from build123d import *

# Parameters (mm, degrees)
BOSS_EXTRUDE1_DEPTH = 114.3
SKETCH6_W           = 27.94
SKETCH6_H           = 30.48
BOSS_EXTRUDE5_DEPTH = 3.81
SKETCH8_W           = 7.62
SKETCH8_H           = 12.7
BOSS_EXTRUDE6_DEPTH = 17.78
SKETCH9_W           = 2.54
SKETCH9_H           = 10.16
BOSS_EXTRUDE7_DEPTH = 114.3
SKETCH10_W          = 2.54
SKETCH10_H          = 2.54
CUT_EXTRUDE2_DEPTH  = 124.399306724
SKETCH11_R          = 0.635
CUT_EXTRUDE3_DEPTH  = 127.822075365
FILLET3_R           = 1.27
FILLET4_R           = 1.27


with BuildPart() as part:
    # Sketch1 → Boss-Extrude1 (new body)
    with BuildSketch(Plane.XY):
        Polygon((27.94, 30.48), (27.94, 27.94), (20.32, 27.94), (20.32, 24.13), (15.24, 24.13), (15.24, 27.94), (7.62, 27.94), (7.62, 24.13), (2.54, 24.13), (2.54, 6.35), (7.62, 6.35), (7.62, 2.54), (15.24, 2.54), (15.24, 6.35), (20.32, 6.35), (20.32, 2.54), (27.94, 2.54), (27.94, 0), (0, 0), (0, 30.48), align=None)
    extrude(amount=BOSS_EXTRUDE1_DEPTH)

    # Sketch6 → Boss-Extrude5 (add)
    with BuildSketch(Plane(origin=(0, 0, 0), x_dir=(-1, 0, 0), z_dir=(0, 0, -1))):
        with Locations((-13.97, 15.24)):
            Rectangle(SKETCH6_W, SKETCH6_H)
    extrude(amount=BOSS_EXTRUDE5_DEPTH)

    # Sketch8 → Boss-Extrude6 (add)
    with BuildSketch(Plane(origin=(27.94, 0, 0), x_dir=(0, 0, -1), z_dir=(1, 0, 0))):
        with Locations((0, 6.35)):
            Rectangle(SKETCH8_W, SKETCH8_H)
    extrude(amount=BOSS_EXTRUDE6_DEPTH)

    # Sketch9 → Boss-Extrude7 (add, through all)
    with BuildSketch(Plane.XY):
        with Locations((26.67, 7.62)):
            Rectangle(SKETCH9_W, SKETCH9_H)
    extrude(amount=BOSS_EXTRUDE7_DEPTH)

    # Sketch10 → Cut-Extrude2 (cut, through all)
    with BuildSketch(Plane.XY.offset(3.81)):
        with Locations((29.21, 11.43)):
            Rectangle(SKETCH10_W, SKETCH10_H)
    extrude(amount=-CUT_EXTRUDE2_DEPTH, mode=Mode.SUBTRACT)

    # Sketch11 → Cut-Extrude3 (cut, through all)
    with BuildSketch(Plane.XY):
        with Locations((10.16, 13.41906471)):
            Circle(SKETCH11_R)
        with Locations((12.7, 13.41906471)):
            Circle(SKETCH11_R)
    extrude(amount=-CUT_EXTRUDE3_DEPTH, mode=Mode.SUBTRACT)

    # Fillet3
    fillet3_edges = [part.edges().sort_by_distance(p)[0] for p in [
        (20.32, 27.94, 57.15),
        (20.32, 24.13, 57.15),
        (15.24, 24.13, 57.15),
        (15.24, 27.94, 57.15),
        (7.62, 27.94, 57.15),
        (7.62, 24.13, 57.15),
        (2.54, 24.13, 57.15),
        (2.54, 6.35, 57.15),
        (7.62, 6.35, 57.15),
        (7.62, 2.54, 57.15),
        (15.24, 2.54, 57.15),
        (15.24, 6.35, 57.15),
        (20.32, 6.35, 57.15),
        (20.32, 2.54, 57.15),
        (25.4, 2.54, 57.15),
    ]]
    fillet(fillet3_edges, radius=FILLET3_R)

    # Fillet4
    fillet4_edges = [part.edges().sort_by_distance(p)[0] for p in [
        (45.72, 0, 0),
        (45.72, 12.7, 0),
    ]]
    fillet(fillet4_edges, radius=FILLET4_R)


solid = part.part
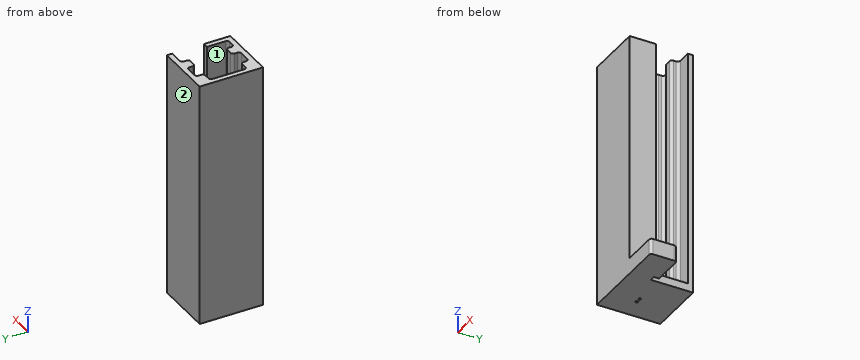
Could you check a few things on this model? Use its own coordinates, in mm. Face numbers are marked on the shaded views. A direction names the side the tool comes from. Give positions to 0.01 mm unless a question says otherwise; leave off trailing zeros. Loops run counter-clockwise (first coordinate to the right, second up) from the corner with the lowest first, then second, coordinate; pieces in that order, holes last. Notation, with made-up numbers: (5, 81.5) -> (52, 81.5) arc R30 ccw to (52, 103.5) -> close; hole circle Ø2 at (51, 67). An arc over 180 degrees is marked (long way). Answer as CSV lines item,"result". Start each with the question number.
(1) If we section it at B-B on x = 35.5: Write out the boundary of the cut face in (y, z).
(2) I'm going to push flat-ended pins straight in: pin 1 Ø2.5 at (x, z) = (35.5, -0.5) entering from +Y; pin 2 Ø10 at (y, z) = (10, 64) entering from +X; pin 3 Ø1 at (y, z) = (21, 84) entering from +X. Where does each tip first touch, or does it pass through?
(3) If we section it at A-A on y = 9: Write out the boundary of the cut face in (x, z), then the cut area to 3 significant figures.
(4) I need wall thicknesses on probe 1 along X at (y, z) = (4.5, 87.5); probe 2 along X at (y, z) = (25.5, 70.5); probe 3 along Y at (x, z) = (13.5, 65.5). Which ranges of each line are inside material? Lowest first, please.
(5) Which directions (+Z, -Z, +X, -X, +Y, -Y) give clear straight access to the entire face, cutting with the end or side of a thin tool? Please do the marked faces 1 and 2.
Computed:
1,outline,"(0, -3.81) -> (12.7, -3.81) -> (12.7, 3.81) -> (0, 3.81) -> close"
2,pin 1,"stops at y = 12.7"
2,pin 2,"stops at x = 27.94"
2,pin 3,"stops at x = 2.54"
3,outline,"(0, -3.81) -> (45.72, -3.81) -> (45.72, 3.81) -> (27.94, 3.81) -> (27.94, 114.3) -> (25.4, 114.3) -> (25.4, 0) -> (2.54, 0) -> (2.54, 114.3) -> (0, 114.3) -> close"
3,area,"823 mm2"
4,probe 1,"x = 0 to 7.62, 15.24 to 20.32, 25.4 to 27.94"
4,probe 2,"x = 0 to 7.62, 15.24 to 20.32"
4,probe 3,"y = 0 to 2.54, 27.94 to 30.48"
5,face 1,"+Z"
5,face 2,"+Z, -Z, +X, -X, +Y"
